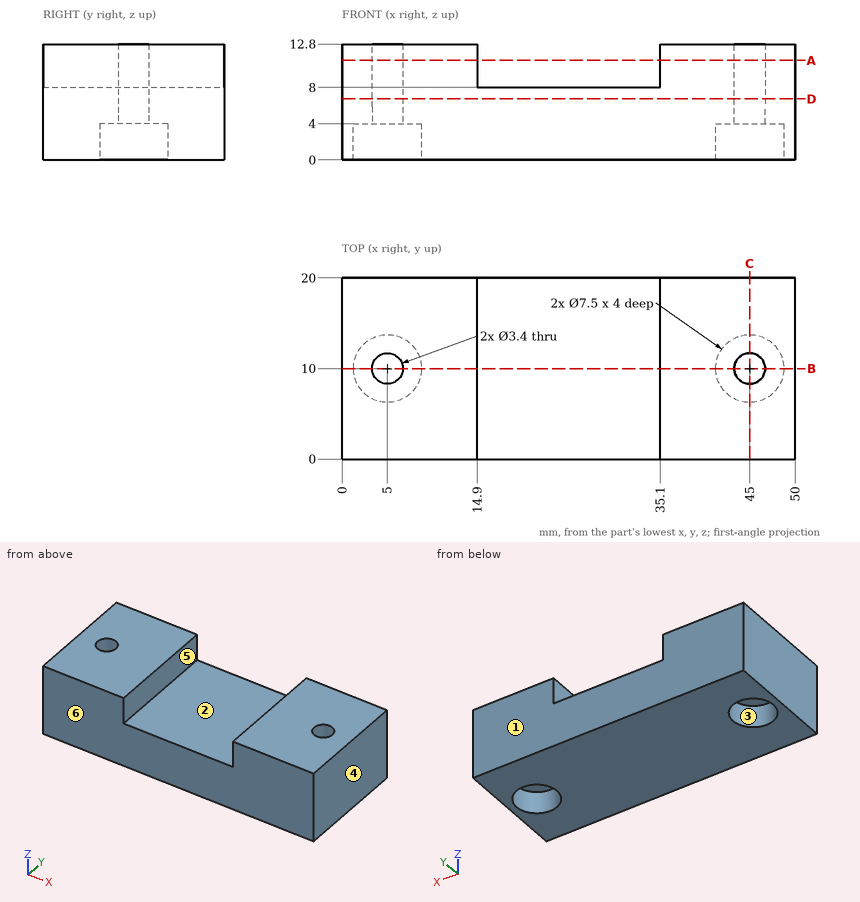
The drawing under review shows one solid part. Ordinate dimensions are in mm from its lowest x, y, z. A direction names the side the tool comes from. Give positions to 0.01 mm unless a question says otherwise; leave off trailing zeros. Order: outer loops, then holes, each group sorted by start corner. A loop starts at its lowest first (then second) coordinate and runs counter-clockwise, first axis right, second up. Notation, with made-up numbers: (26.25, 23) -> (37.25, 23) arc R25 ccw to (37.25, 48) -> close; hole circle Ø2 at (66.5, 30.25). An arc over 180 degrees is marked (long way). Write item = value, one per line.
1) Draft analysis for pull direction X (two halves, no side actions). For the marked faces 4, 5 and 6, state which applies: pulls with the +X half, pulls with the -X half, needs draft (parallel to the pull), parting line crosses it, or undercut.
Findings:
face_4 = pulls with the +X half
face_5 = undercut
face_6 = needs draft
2) Insertion check: pin 1 (6 mm diameter, centred on x = 4, y = 12, fed in from -Z); pin 2 (5 mm diameter, centred on x = 18, y = 16, fed in from +Z); pin 3 (3 mm diameter, centred on x = 45, y = 10, fed in from -Z); pin 4 (5.5 mm diameter, centred on x = 5, y = 10, fed in from -Z). Each pin has a flat end and moves straight along its axis. Give the tip position at first contact, or say it passes through.
Findings:
pin_1 = 0
pin_2 = 8
pin_3 = through
pin_4 = 4
3) We need section D-D, the plane z = 6.75. Give the boundary of the cut face in (x, y).
Findings:
outline = (0, 0) -> (50, 0) -> (50, 20) -> (0, 20) -> close; hole circle Ø3.4 at (5, 10); hole circle Ø3.4 at (45, 10)
4) To check wall thickness, follow L1, parallel to Y at x = 5, z = 5.1; L2, parallel to X at y = 8.25, z = 3.5; L3, parallel to X at y = 10, z = 10.75. State the ranges of each line that lie inside material, in increasing order. Write a range as from..to.
Findings:
L1 = 0..8.3, 11.7..20
L2 = 0..1.68, 8.32..41.68, 48.32..50
L3 = 0..3.3, 6.7..14.9, 35.1..43.3, 46.7..50
5) For the marked faces 1, 2 and 3, list the 3-axis set-ups (+Z, -Z, +X, -X, +Y, -Y) from which the entire face can be reached by the end or side of a thin tool; tool diameter is ignored.
Findings:
face_1 = +Z, -Z, +X, -X, +Y
face_2 = +Z, +Y, -Y
face_3 = -Z
6) We need section C-C, the plane x = 45. Give the boundary of the cut face in (y, z), and give its area (3 significant figures).
Findings:
outline = (0, 0) -> (6.25, 0) -> (6.25, 4) -> (8.3, 4) -> (8.3, 12.8) -> (0, 12.8) -> close; (11.7, 4) -> (13.75, 4) -> (13.75, 0) -> (20, 0) -> (20, 12.8) -> (11.7, 12.8) -> close
area = 196 mm^2
7) We need section A-A, the plane z = 11. Give the boundary of the cut face in (x, y).
Findings:
outline = (0, 0) -> (14.9, 0) -> (14.9, 20) -> (0, 20) -> close; (35.1, 0) -> (50, 0) -> (50, 20) -> (35.1, 20) -> close; hole circle Ø3.4 at (5, 10); hole circle Ø3.4 at (45, 10)
8) We need section B-B, the plane y = 10. Give the boundary of the cut face in (x, z), and give its area (3 significant figures).
Findings:
outline = (0, 0) -> (1.25, 0) -> (1.25, 4) -> (3.3, 4) -> (3.3, 12.8) -> (0, 12.8) -> close; (6.7, 4) -> (8.75, 4) -> (8.75, 0) -> (41.25, 0) -> (41.25, 4) -> (43.3, 4) -> (43.3, 12.8) -> (35.1, 12.8) -> (35.1, 8) -> (14.9, 8) -> (14.9, 12.8) -> (6.7, 12.8) -> close; (46.7, 4) -> (48.75, 4) -> (48.75, 0) -> (50, 0) -> (50, 12.8) -> (46.7, 12.8) -> close
area = 423 mm^2
